Read the model definition and answer for the solid it produces. Units are mm, in the model's axes. A direction names the side the tool comes from. Coordinates: 2 decimals unless noted, no trailing zeros. Loops run counter-clockwise (first coordinate to the right, second up) from the corner with the lowest first, then second, coordinate; pieces in that order, holes last. Notation, with made-up numbers: (-28.5, -12.75) - (26.5, -12.75) arc R11 ccw to (26.5, -7.75) - close; hole circle Ø3 at (-12.75, 27.5). An arc over 180 degrees is marked (long way). Use one line per item in the form item = value.
Autodesk Inventor part; units mm, degrees
ref_plane "YZ Plane" through (0, 0, 0) normal (1, 0, 0) x (0, 1, 0)
ref_plane "XZ Plane" through (0, 0, 0) normal (0, 1, 0) x (-1, 0, 0)
ref_plane "XY Plane" through (0, 0, 0) normal (0, 0, 1) x (1, 0, 0)
sketch "Эскиз8" plane through (0, 0, 0) normal (0, 0, 1) x (1, 0, 0)
  line L0 (-9, -9.9543) -> (-9, 10.0457)
  line L1 (0, 17.0842) -> (0, -16.9927)
  line L2 (0, 16.7842) -> (-3, 16.7842)
  line L3 (-3, 16.7842) -> (-3, -16.6927)
  line L4 (-3, -16.6927) -> (0, -16.6927)
  line L5 (0, -16.6927) -> (0, 16.7842)
  line L6 (-44, 11.5457) -> (-9, 11.5457)
  line L7 (-9, 15.5842) -> (-44, 15.5842)
  line L8 (-44, 15.5842) -> (-44, 11.5457)
  line L9 (-44, -15.4927) -> (-9, -15.4927)
  line L10 (-9, -11.4543) -> (-44, -11.4543)
  line L11 (-44, -11.4543) -> (-44, -15.4927)
  line L12 (-9, 15.2842) -> (-44, 15.2842)
  line L13 (-44, -15.1927) -> (-9, -15.1927)
  line L14 (-44, 11.8457) -> (-9.3, 11.8457)
  line L15 (-44, -11.7543) -> (-9.3, -11.7543)
  line L16 (-9.3, 15.2842) -> (-3, 15.2842)
  line L17 (-3, 15.2842) -> (-3, 11.8457)
  line L18 (-3, 11.8457) -> (-9.3, 11.8457)
  line L19 (-9.3, -11.7543) -> (-3, -11.7543)
  line L20 (-3, -11.7543) -> (-3, -15.1927)
  line L21 (-3, -15.1927) -> (-9.3, -15.1927)
  line L22 (-37.3, 15.2842) -> (-37.3, -15.1927)
  arc A0 (-10.5, -11.4543) -> (-9, -9.9543) centre (-10.5, -9.9543) ccw
  arc A1 (-9, 10.0457) -> (-10.5, 11.5457) centre (-10.5, 10.0457) ccw
  line L23 (-10.5, 11.5457) -> (-32.1754, 11.5457)
  line L24 (-32.1754, 11.5457) -> (-31.4296, 7.5457)
  line L25 (-31.4296, 7.5457) -> (-26.1754, 7.5457)
  line L26 (-26.1754, -4.9543) -> (-26.1754, -7.4543)
  line L27 (-25.1754, 4.0457) -> (-24.6192, 4.0457)
  line L28 (-24.6192, 4.0457) -> (-24.6192, 9.5457)
  spline S0 degree 3 poles (-24.1006, 10.0457) (-24.1642, 10.0457) (-24.2391, 10.0312) (-24.3567, 9.984) (-24.4205, 9.943) (-24.5115, 9.8556) (-24.5549, 9.7937) (-24.6042, 9.6794) (-24.6192, 9.6072) (-24.6192, 9.5457) knots 0.074888 0.074888 0.074888 0.074888 0.093967 0.093967 0.112918 0.112918 0.131824 0.131824 0.15026 0.15026 0.15026 0.15026
  line L29 (-24.1006, 10.0457) -> (-24.0379, 10.0457)
  spline S1 degree 3 poles (-23.5192, 9.5457) (-23.5192, 9.6072) (-23.5343, 9.6794) (-23.5836, 9.7937) (-23.6269, 9.8556) (-23.718, 9.943) (-23.7817, 9.984) (-23.8994, 10.0312) (-23.9743, 10.0457) (-24.0379, 10.0457) knots 0.15026 0.15026 0.15026 0.15026 0.168696 0.168696 0.187602 0.187602 0.206553 0.206553 0.225632 0.225632 0.225632 0.225632
  line L30 (-23.5192, 9.5457) -> (-23.5192, 4.0457)
  line L31 (-22.8192, 4.0457) -> (-22.8192, -3.9543)
  line L32 (-22.8192, -3.9543) -> (-23.5192, -3.9543)
  line L33 (-23.5192, -3.9543) -> (-23.5192, -9.4543)
  spline S2 degree 3 poles (-24.0379, -9.9543) (-23.9743, -9.9543) (-23.8994, -9.9398) (-23.7817, -9.8925) (-23.718, -9.8516) (-23.6269, -9.7642) (-23.5836, -9.7022) (-23.5343, -9.5879) (-23.5192, -9.5157) (-23.5192, -9.4543) knots 0.074888 0.074888 0.074888 0.074888 0.093967 0.093967 0.112918 0.112918 0.131824 0.131824 0.15026 0.15026 0.15026 0.15026
  line L34 (-24.0379, -9.9543) -> (-24.1006, -9.9543)
  spline S3 degree 3 poles (-24.6192, -9.4543) (-24.6192, -9.5157) (-24.6042, -9.5879) (-24.5549, -9.7022) (-24.5115, -9.7642) (-24.4205, -9.8516) (-24.3567, -9.8925) (-24.2391, -9.9398) (-24.1642, -9.9543) (-24.1006, -9.9543) knots 0.15026 0.15026 0.15026 0.15026 0.168696 0.168696 0.187602 0.187602 0.206553 0.206553 0.225632 0.225632 0.225632 0.225632
  line L35 (-24.6192, -9.4543) -> (-24.6192, -3.9543)
  line L36 (-24.6192, -3.9543) -> (-25.1754, -3.9543)
  line L37 (-26.1754, 7.5457) -> (-26.1754, 5.0457)
  line L38 (-26.1754, -7.4543) -> (-31.4296, -7.4543)
  line L39 (-31.4296, -7.4543) -> (-32.1754, -11.4543)
  line L40 (-32.1754, -11.4543) -> (-10.5, -11.4543)
  line L41 (-26.1754, -4.9543) -> (-25.1754, -3.9543)
  line L42 (-25.1754, 4.0457) -> (-26.1754, 5.0457)
  line L43 (-23.5192, 4.0457) -> (-22.8192, 4.0457)
  point P0 (0, 0)
  point P1 (-32.1754, 15.5842)
  point P2 (-32.1754, -15.4927)
  point P3 (0, -16.6927)
  point P4 (-3, 15.2842)
  point P5 (-37.3, 11.8457)
  point P6 (-9.3, 11.8457)
  point P7 (-37.3, -11.7543)
  point P8 (-9, -15.1927)
  dimension "d40" = 3
  dimension "d43" = 0.3
  dimension "d44" = 0.3
  dimension "d45" = 0.3
  dimension "d46" = 0.3
  dimension "d47" = 6.7
extrude "Выдавливание8" add sketch "Эскиз8" against normal blind 1.9 contours L15 L19 L3 L21 L13 L22 | L22 L12 L16 L3 L18 L14 | L3 L2 L1 L4
sketch "Эскиз9" plane through (0, 0, -1.9) normal (0, 0, -1) x (-1, 0, 0)
  line L0 (0, 16.7842) -> (0, -16.6927)
  line L1 (0, -16.6927) -> (3, -16.6927)
  line L2 (3, -16.6927) -> (3, -15.1927)
  line L3 (3, -15.1927) -> (37.3, -15.1927)
  line L4 (37.3, -15.1927) -> (37.3, -11.7543)
  line L5 (37.3, -11.7543) -> (3, -11.7543)
  line L6 (3, -11.7543) -> (3, 11.8457)
  line L7 (3, 11.8457) -> (37.3, 11.8457)
  line L8 (37.3, 11.8457) -> (37.3, 15.2842)
  line L9 (37.3, 15.2842) -> (3, 15.2842)
  line L10 (3, 15.2842) -> (3, 16.7842)
  line L11 (3, 16.7842) -> (0, 16.7842)
  line L12 (37.3, 15.2842) -> (3, 15.2842)
  line L13 (3, -15.1927) -> (37.3, -15.1927)
  line L14 (3, 15.2842) -> (3, -15.1927)
  point P0 (0, 0)
  point P1 (3, -11.7543)
extrude "Выдавливание9" add sketch "Эскиз9" along normal blind 3.5 contours L11 L10 L14 L6 L2 L1 L0
fillet "Сопряжение9" radius 1.5 4 edges at (-3, 15.2842, -0.95) (-3, 11.8457, -0.95) (-3, -11.7543, -0.95) (-3, -15.1927, -0.95)
sketch "Эскиз10" plane through (-3, -16.6927, -5.4) normal (-1, 0, 0) x (0, 0, 1)
  arc A0 (1.4727, 14.8527) -> (1.4727, 18.6243) centre (2.7, 16.7385) ccw
  circle A1 centre (2.7, 16.7385) radius 2.25
  point P0 (5.4, 16.6927)
  point P1 (1.4727, 18.6243)
extrude "Выдавливание10" cut sketch "Эскиз10" against normal blind 1.5
sketch "Эскиз11" plane through (-3, -16.6927, -5.4) normal (-1, 0, 0) x (0, 0, 1)
  point P0 (5.4, 16.6927)
sketch "Эскиз12" plane through (-3, -16.6927, -5.4) normal (-1, 0, 0) x (0, 0, 1)
  circle A0 centre (2.7, 16.7385) radius 2.25
  line L0 (3.5, 6.4385) -> (3.5, 0)
  line L1 (5.4, 6.4385) -> (3.5, 6.4385)
  line L2 (5.4, 27.0385) -> (5.4, 6.4385)
  line L3 (3.5, 27.0385) -> (5.4, 27.0385)
  line L4 (3.5, 33.4769) -> (3.5, 27.0385)
  line L5 (3.5, 33.4769) -> (0, 33.4769)
  line L6 (0, 0) -> (0, 33.4769)
  line L7 (3.5, 0) -> (0, 0)
  line L8 (3.5, 1.5) -> (3.5, 0)
  line L9 (5.4, 0) -> (3.5, 0)
  line L10 (5.4, 0) -> (5.4, 1.5)
  line L11 (5.4, 1.5) -> (3.5, 1.5)
  line L12 (5.4, 33.4769) -> (0, 33.4769)
  line L13 (5.4, 0) -> (3.5, 0)
  line L14 (3.5, 0) -> (3.5, -2)
  line L15 (3.5, -2) -> (5.4, -2)
  line L16 (5.4, -2) -> (5.4, 0)
  line L17 (3.5, 6.4385) -> (3.5, 0)
  line L18 (5.4, 33.4769) -> (3.5, 33.4769)
  line L19 (5.4, 33.4769) -> (3.5, 33.4769)
  line L20 (3.5, 33.4769) -> (3.5, 35.4769)
  line L21 (3.5, 35.4769) -> (5.4, 35.4769)
  line L22 (5.4, 35.4769) -> (5.4, 33.4769)
  line L23 (3.5, 33.4769) -> (3.5, 27.0385)
  point P0 (5.4, 16.6927)
  dimension "d56" = 2
  dimension "d57" = 2
extrude "Выдавливание11" add sketch "Эскиз12" against normal blind 1.5 contours L20 L21 L22 L12 | L9 L16 L15 L14
sketch "Эскиз13" plane through (-37.3, 15.2842, 0) normal (0, 1, 0) x (1, 0, 0)
  line L0 (32.8, 1.9) -> (32.8, 0)
  line L1 (0, 1.9) -> (32.8, 1.9)
  line L2 (0, 0) -> (0, 1.9)
  line L3 (32.8, 0) -> (0, 0)
  circle A0 centre (1, 0.75) radius 0.5
  circle A1 centre (1, 0.75) radius 0.75
  line L4 (1, 0.75) -> (0, 0.75)
  point P0 (37.3, 0)
  dimension "d60" = 1
  dimension "d61" = 1.5
  dimension "d62" = 1
extrude "Выдавливание12" cut sketch "Эскиз13" against normal blind 40 contours A0
properties part number "motherboard_key"
Item 1: The part is cut by section B-B on y = 13. Give the vertices of the cut face in (x, z).
Results below:
outline = (-37.3, -1.9) - (-3, -1.9) - (-3, -5.4) - (0, -5.4) - (0, 0) - (-37.3, 0) - close; hole circle Ø1 at (-36.3, -0.75)
Item 2: For a pull along Y with two mould halves and no side action, classify faces 4 (the flat face through (-21, 15.284, -1)), 5 (the flat face through (-20, 14, -1.9)), 6 (the cylindrical face through (-3.428, -11.303, -0.963)) as +Y half, -Y half, draft (parallel to the pull), parting line (faces both ways), or undercut.
Results below:
face_4 = +Y half
face_5 = draft
face_6 = undercut
Item 3: Which of the six approach directions +Z, -Z, +X, -X, +Y, -Y give full straight-line access (tool end or side, diameter ignored) to faces 1 (the flat face through (-3, -0.2, -5.1)), 2 (the flat face through (-2, -18, -1.9)), 3 (the flat face through (-21, 11.846, -1))?
Results below:
face_1 = -Z, -X
face_2 = -Z, +X, -X, -Y
face_3 = +Z, -Z, -X
Item 4: The part is cut by section C-C on x = -20.5. Give the vertices of the cut face in (y, z), plus the area to 3 significant figures.
Results below:
outline = (-15.19, -1.9) - (-11.75, -1.9) - (-11.75, 0) - (-15.19, 0) - close; (11.85, -1.9) - (15.28, -1.9) - (15.28, 0) - (11.85, 0) - close
area = 13.1 mm²
Item 5: The part is cut by section D-D on z = -2.7. Give the vertices of the cut face in (x, y).
Results below:
outline = (-3, -16.69) - (0, -16.69) - (0, 16.78) - (-3, 16.78) - (-3, 2.3) - (-1.5, 2.3) - (-1.5, -2.2) - (-3, -2.2) - close
Item 6: The part is cut by section A-A on x = -36.3. Give the vertices of the cut face in (y, z), plus the area to 3 significant figures.
Results below:
outline = (-15.19, -1.9) - (-11.75, -1.9) - (-11.75, -1.25) - (-15.19, -1.25) - close; (-15.19, -0.25) - (-11.75, -0.25) - (-11.75, 0) - (-15.19, 0) - close; (11.85, -1.9) - (15.28, -1.9) - (15.28, -1.25) - (11.85, -1.25) - close; (11.85, -0.25) - (15.28, -0.25) - (15.28, 0) - (11.85, 0) - close
area = 6.19 mm²
Item 7: Find the intervals of material crossed by L1, parallel to Z at x = -36.3, y = -12.4; L2, parallel to Y at x = -2.35, z = -2.7; L3, parallel to X at y = 12.8, z = -0.75, in increasing order.
Results below:
L1 = -1.9 to -1.25, -0.25 to 0
L2 = -16.69 to -2.2, 2.3 to 16.78
L3 = -37.3 to -36.8, -35.8 to 0
Item 8: Each of these flat-tipped pins is pushed along its axis until it touches: P1, Ø0.6, axis at x = -25.5, z = -0.5, coming from the -Y side; P2, Ø2.5, axis at y = 0.5, z = -3, coming from the -X side; P3, Ø0.9, axis at x = -1.5, z = -3.5, coming from the -Y side; P4, Ø12, axis at x = -10.5, y = -10.5, coming from the +Z side. Where does it stop, or does it pass through?
Results below:
P1 = -15.19
P2 = -1.5
P3 = -16.69
P4 = 0
